from build123d import *

# Parameters (mm, degrees)
SKETCH_1_W          = 42
SKETCH_1_H          = 42
SKETCH_1_R          = 1.7
EXTRUDE_1_DEPTH     = 8
CHAMFER_1_SIZE      = 5
CUT_EXTRUDE_1_DEPTH = 5
SKETCH_3_R          = 1.7
EXTRUDE_2_DEPTH     = 2
SKETCH_4_R          = 3.2
CUT_EXTRUDE_2_DEPTH = 2.4
SKETCH_5_R          = 3.4
CUT_EXTRUDE_3_DEPTH = 2.4
FILLET_1_R          = 1


with BuildPart() as part:
    # Эскиз1 → Бобышка-Вытянуть1 (new body)
    with BuildSketch(Plane.XY):
        Rectangle(SKETCH_1_W, SKETCH_1_H)
        with Locations((-15.5, -15.5)):
            Circle(SKETCH_1_R, mode=Mode.SUBTRACT)
        with Locations((-15.5, 15.5)):
            Circle(SKETCH_1_R, mode=Mode.SUBTRACT)
        with Locations((15.5, 15.5)):
            Circle(SKETCH_1_R, mode=Mode.SUBTRACT)
        with BuildLine():
            Line((0, -8), (-10, -8))
            ThreePointArc((-10, -8), (-18, 0), (-10, 8))
            Line((-10, 8), (0, 8))
            ThreePointArc((0, 8), (8, 0), (0, -8))
        make_face(mode=Mode.SUBTRACT)
    extrude(amount=EXTRUDE_1_DEPTH)

    # Фаска1
    chamfer_1_edges = [part.edges().sort_by_distance(p)[0] for p in [
        (-21, 21, 4),
        (21, 21, 4),
        (21, -21, 4),
        (-21, -21, 4),
    ]]
    chamfer(chamfer_1_edges, length=CHAMFER_1_SIZE)

    # Эскиз2 → Вырез-Вытянуть1 (cut)
    with BuildSketch(Plane.XY.offset(8)):
        with BuildLine():
            Line((-10.5, 15.5), (-10.5, 19))
            Line((-10.5, 19), (10.5, 19))
            Line((10.5, 19), (10.5, 15.5))
            ThreePointArc((10.5, 15.5), (11.964466094, 11.964466094), (15.5, 10.5))
            Line((15.5, 10.5), (19, 10.5))
            Line((19, 10.5), (19, -10))
            ThreePointArc((19, -10), (16.363961031, -16.363961031), (10, -19))
            Line((10, -19), (-10.5, -19))
            Line((-10.5, -19), (-10.5, -15.5))
            ThreePointArc((-10.5, -15.5), (-11.964466094, -11.964466094), (-15.5, -10.5))
            Line((-15.5, -10.5), (-19, -10.5))
            Line((-19, -10.5), (-19, 10.5))
            Line((-19, 10.5), (-15.5, 10.5))
            ThreePointArc((-15.5, 10.5), (-11.964466094, 11.964466094), (-10.5, 15.5))
        make_face()
    extrude(amount=-CUT_EXTRUDE_1_DEPTH, mode=Mode.SUBTRACT)

    # Эскиз3 → Бобышка-Вытянуть2 (add)
    with BuildSketch(Plane.XY.offset(8)):
        with BuildLine():
            Line((-20.370828693, -16.629171307), (-16.629171307, -20.370828693))
            ThreePointArc((-16.629171307, -20.370828693), (-11.964466094, -11.964466094), (-20.370828693, -16.629171307))
        make_face()
        with Locations((-15.5, -15.5)):
            Circle(SKETCH_3_R, mode=Mode.SUBTRACT)
    extrude(amount=EXTRUDE_2_DEPTH)

    # Эскиз4 → Вырез-Вытянуть2 (cut)
    with BuildSketch(Plane.XY.offset(8)):
        with Locations((-15.5, 15.5)):
            Circle(SKETCH_4_R)
        with Locations((15.5, 15.5)):
            Circle(SKETCH_4_R)
    extrude(amount=-CUT_EXTRUDE_2_DEPTH, mode=Mode.SUBTRACT)

    # Эскиз5 → Вырез-Вытянуть3 (cut)
    with BuildSketch(Plane(origin=(0, 0, 0), x_dir=(-1, 0, 0), z_dir=(0, 0, -1))):
        with Locations((-15.5, 15.5)):
            Circle(SKETCH_5_R)
        with Locations((15.5, 15.5)):
            Circle(SKETCH_5_R)
        with Locations((15.5, -15.5)):
            Circle(SKETCH_5_R)
    extrude(amount=-CUT_EXTRUDE_3_DEPTH, mode=Mode.SUBTRACT)

    # Скругление1
    fillet_1_edges = [part.edges().sort_by_distance(p)[0] for p in [
        (-10.5, 19, 5.5),
        (10.5, 19, 5.5),
        (19, 10.5, 5.5),
        (-10.5, -19, 5.5),
        (-19, -10.5, 5.5),
        (-19, 10.5, 5.5),
    ]]
    fillet(fillet_1_edges, radius=FILLET_1_R)


solid = part.part
The model under review builds one solid part; all positions refer to its coordinate system, in mm. A direction names the side the tool comes from. Round coordinates to 2 decimals unless told otherwise and drop trailing zeros. Loops run counter-clockwise (first coordinate to the right, second up) from the corner with the lowest first, then second, coordinate; pieces in that order, holes last. Notation, with made-up numbers: (-30.75, 3.5) -> (8.25, 3.5) arc R23 ccw to (8.25, 26.5) -> close; hole circle Ø10 at (46, -22). An arc over 180 degrees is marked (long way). Answer as CSV lines item,"result".
1) For P1, Ø8, axis at x = 8.5, y = -2, coming from the +Z side; P2, Ø4, axis at x = -15.5, y = -15.5, coming from the -Z side; P3, Ø4.5, axis at x = -15.5, y = 15.5, coming from the +Z side; P4, Ø3, axis at x = -15.5, y = -15.5, coming from the +Z side (3 decimals), all flat-tipped, find the tip position at first contact; note any pin that passes through.
Geometry results:
P1,"stops at z = 3"
P2,"stops at z = 2.4"
P3,"stops at z = 5.6"
P4,"passes through"
2) Add section D-D on z = 8.75. Write out the cut boundary in (x, y).
Geometry results:
outline,"(-20.37, -16.63) -> (-16.63, -20.37) arc R5 ccw (long way) to start; hole circle Ø3.4 at (-15.5, -15.5)"
3) Add section A-A on x = -9. Write out the cut boundary in (y, z), plus the area to 3 significant figures.
Geometry results:
outline,"(-21, 0) -> (-8, 0) -> (-8, 3) -> (-19, 3) -> (-19, 8) -> (-21, 8) -> close; (8, 0) -> (21, 0) -> (21, 8) -> (19, 8) -> (19, 3) -> (8, 3) -> close"
area,"98.0 mm²"
4) Draft analysis for pull direction Y (two halves, no side actions). For faces 1 (the face through (17, 10.5, 6)), 2 (the face through (19, 18, 4)), 3 (the face through (21, 0, 4)), state which applies: pulls with the +Y half, pulls with the -Y half, needs draft (parallel to the pull), parting line crosses it, or undercut.
Geometry results:
face 1,"undercut"
face 2,"pulls with the +Y half"
face 3,"needs draft"
5) To check wall thickness, follow line 1 along Y through (x, z) = (-4, 6); line 2 along X through (y, z) = (17.5, 0.5); line 3 along Y through (x, z) = (15.5, 1.65). State the ranges of each line that lie inside material, in increasing order. Write a range as from..to.
Geometry results:
line 1,"y = -21..-19, 19..21"
line 2,"x = -19.5..-18.25, -12.75..12.75, 18.25..19.5"
line 3,"y = -21..12.1, 18.9..21"
6) Add section C-C on y = 0. Write out the cut boundary in (x, z).
Geometry results:
outline,"(-21, 0) -> (-18, 0) -> (-18, 3) -> (-19, 3) -> (-19, 8) -> (-21, 8) -> close; (8, 0) -> (21, 0) -> (21, 8) -> (19, 8) -> (19, 3) -> (8, 3) -> close"
7) Tool access review of faces 4 (the face through (-5, -8, 1)), 5 (the face through (0, -21, 4)), 6 (the face through (14, 14, 2.4)), 7 (the face through (-18.715, 10.199, 5.465)): name each direction out of +Z, -Z, +X, -X, +Y, -Y from which nothing blocks a thin tool from reaching the whole face with its end or side.
Geometry results:
face 4,"+Z, -Z"
face 5,"+Z, -Z, +X, -X, -Y"
face 6,"-Z"
face 7,"+Z"
8) Add section B-B on z = 3.75. State how many separate pieces and enclosed holes the cut face has, plus the area to 3 significant figures.
Geometry results:
separate pieces,"1"
enclosed holes,"4"
area,"462 mm²"
